Verification items for this drawing (mm, ordinates from the low corner). A direction names the side the tool comes from. Round coordinates to 2 decimals unless told otherwise and drop trailing zeros. Loops run counter-clockwise (first coordinate to the right, second up) from the corner with the lowest first, then second, coordinate; pieces in that order, holes last. Notation, with made-up numbers: (-19, 22.25) -> (26, 22.25) arc R21 ccw to (26, 57.25) -> close; hole circle Ø7 at (72, 59.25). An arc over 180 degrees is marked (long way). Use a Markdown table: item, result. Add a question column.
Q1. Sectioned sample at C-C, the plane y = 3. Enter the section's corners in (x, z).
Q2. Set-up check for the marked faces 4, 5 and 6: record each of +Z, -Z, +X, -X, +Y, -Y from which the full face is reachable in a straight line by a thin tool's end or side.
Q3. Material ranges on L1, parallel to Z at x = 1.15, y = 3.65; L2, parallel to Z at x = 1.05, y = 3.2; L3, parallel to X at y = 2, z = 4.05, recorded low to high.
Q4. Sectioned sample at A-A, the plane y = 3.5. Enter the section's corners in (x, z).
Q5. Sectioned sample at D-D, the plane z = 0.9. Enter the section's corners in (x, y).
Q6. Gauge pin test, flat ends, axial feed: P1, Ø1.5, axis at y = 3.5, z = 4, coming from the +X side; P2, Ø2, axis at x = 3, z = 2.5, coming from the +Y side; P3, Ø1.2, axis at y = 0.5, z = 4.5, coming from the -X side. Record the tip position at first contact, or that the pin passes through.
Q7. Sectioned sample at B-B, the plane x = 2.55. Enter the section's corners in (y, z).
Q8. Release check for a two-part mould opening along Z. For the marked faces 1, 2 and 3 record: released by +Z, released by -Z, zero draft, split by the parting line, or undercut.
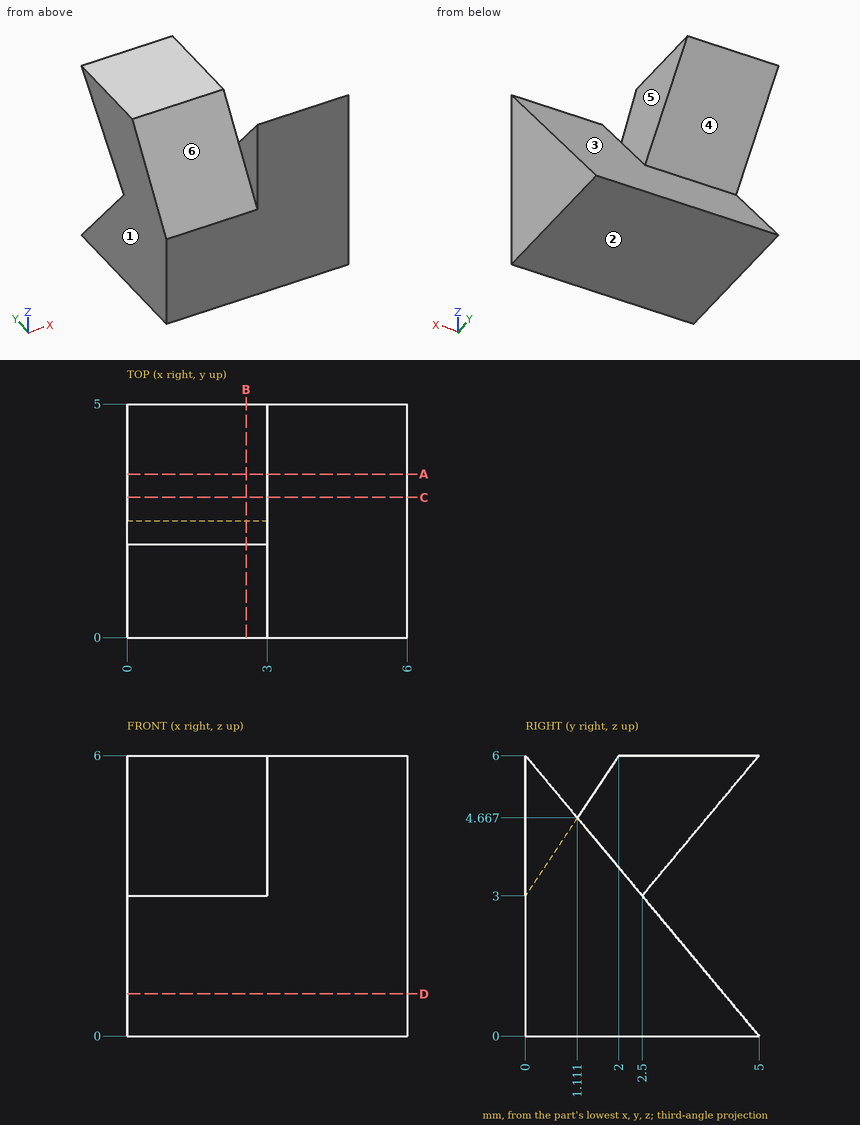
Values:
| question | item | result |
|---|---|---|
| 1 | outline | (0, 0) -> (6, 0) -> (6, 2.4) -> (0, 2.4) -> close; (0, 3.6) -> (3, 3.6) -> (3, 6) -> (0, 6) -> close |
| 2 | face 4 | +X, -X, +Y |
| 2 | face 5 | +Z, +X, +Y |
| 2 | face 6 | +Z, -X, -Y |
| 3 | L1 | 0 to 1.62, 4.38 to 6 |
| 3 | L2 | 0 to 2.16, 3.84 to 6 |
| 3 | L3 | 0 to 3 |
| 4 | outline | (0, 0) -> (6, 0) -> (6, 1.8) -> (0, 1.8) -> close; (0, 4.2) -> (3, 4.2) -> (3, 6) -> (0, 6) -> close |
| 5 | outline | (0, 0) -> (6, 0) -> (6, 4.25) -> (0, 4.25) -> close |
| 6 | P1 | x = 3 |
| 6 | P2 | y = 3.75 |
| 6 | P3 | x = 0 |
| 7 | outline | (0, 0) -> (5, 0) -> (2.5, 3) -> (5, 6) -> (2, 6) -> (0, 3) -> close |
| 8 | face 1 | zero draft |
| 8 | face 2 | released by -Z |
| 8 | face 3 | undercut |
